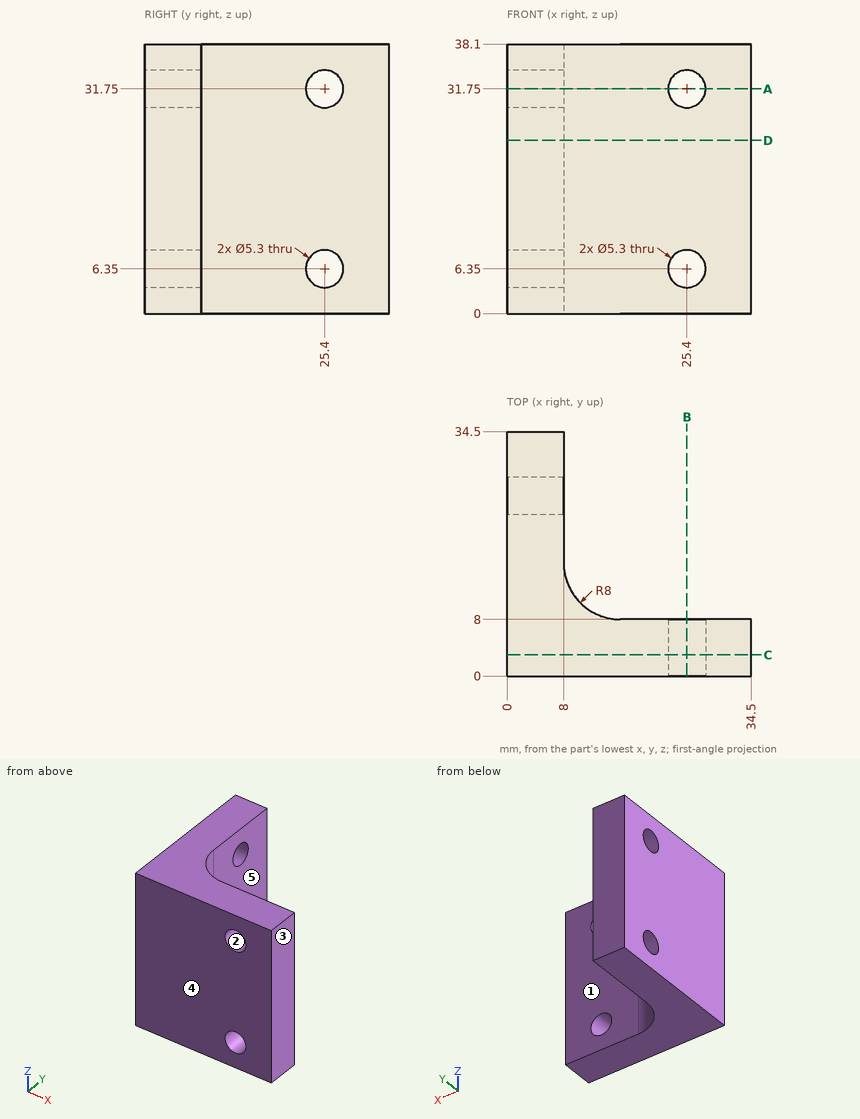
Job drawing, mm, ordinate dimensions from the low corner. One solid piece. A direction names the side the tool comes from. Give positions to 0.01 mm unless a question says otherwise; leave off trailing zeros. Loops run counter-clockwise (first coordinate to the right, second up) from the corner with the lowest first, then second, coordinate; pieces in that order, holes last. Notation, with made-up numbers: M 68,78.25 L 126,78.25 A19 cw 126,93.25 Z; hole C -1,-18.5 d3. An arc over 180 degrees is marked long. Put each result on its own line as item: value. Start each with the question number.
1) Saw through at C-C (y = 3). List the corners of the cut face in (x, z), then the cut area to 3 significant figures.
2) Flat gauge pins, fed straight in: pin 1 (1 mm diameter, centred on x = 29, z = 5, fed in from +Y); pin 2 (3 mm diameter, centred on y = 26.5, z = 21.5, fed in from +X). Where does each tip first touch, or does it go through?
3) Saw through at D-D (z = 24.5). List the corners of the cut face in (x, y), then the cut area to 3 significant figures.
4) Pull direction X, two halves, no side cores. Call the marked faces 1, 2 and 3: +X half, -X half, draft (parallel to the pull), parting line (faces both ways), or undercut.
5) 3-axis set-ups, long thin cutter, end or side, ignore diameter. For the marked faces 4 and 5: which of +Z, -Z, +X, -X, +Y, -Y reach the whole face in a straight line?
6) Saw through at A-A (z = 31.75). List the corners of the cut face in (x, y), then the cut area to 3 significant figures.
7) Probe probe 1 along Z at (x, y) = (25.4, 2); probe 2 along X at (y, z) = (1.5, 31.75); probe 3 along Y at (x, z) = (30, 29). List the from-to ranges inside material, lowest first.
8) Saw through at B-B (x = 25.4). List the corners of the cut face in (y, z).
Numbers:
1. outline: M 0,0 L 34.5,0 L 34.5,38.1 L 0,38.1 Z; hole C 25.4,6.35 d5.3; hole C 25.4,31.75 d5.3
1. area: 1,270 mm^2
2. pin 1: y = 8
2. pin 2: x = 8
3. outline: M 0,0 L 34.5,0 L 34.5,8 L 16,8 A8 cw 8,16 L 8,34.5 L 0,34.5 Z
3. area: 502 mm^2
4. face 1: draft
4. face 2: undercut
4. face 3: +X half
5. face 4: +Z, -Z, +X, -X, -Y
5. face 5: +Z, -Z, +X, +Y
6. outline: M 0,0 L 22.75,0 L 22.75,8 L 16,8 A8 cw 8,16 L 8,22.75 L 0,22.75 Z; M 0,28.05 L 8,28.05 L 8,34.5 L 0,34.5 Z; M 28.05,0 L 34.5,0 L 34.5,8 L 28.05,8 Z
6. area: 417 mm^2
7. probe 1: 0 to 3.7, 9 to 29.1, 34.4 to 38.1
7. probe 2: 0 to 22.75, 28.05 to 34.5
7. probe 3: 0 to 8
8. outline: M 0,0 L 8,0 L 8,3.7 L 0,3.7 Z; M 0,9 L 8,9 L 8,29.1 L 0,29.1 Z; M 0,34.4 L 8,34.4 L 8,38.1 L 0,38.1 Z
